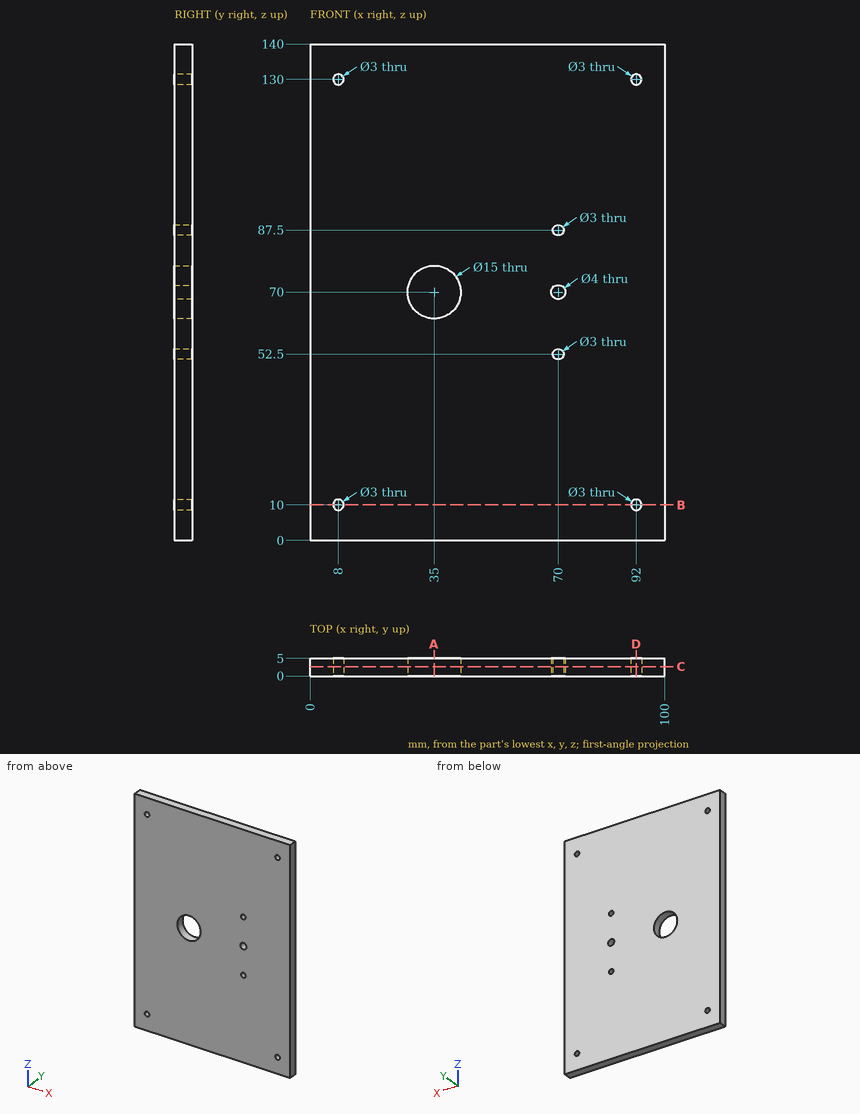
Geometry check sheet. Reference: drawing and pictorial views, mm from the part's lowest x, y, z. Coordinates: 2 decimals unless noted, no trailing zeros. Loops run counter-clockwise (first coordinate to the right, second up) from the corner with the lowest first, then second, coordinate; pieces in that order, holes last.
1) Sectioned sample at B-B (z = 10). Record the boundary of the cut face in (x, y).
2) Sectioned sample at D-D (x = 92). Record the boundary of the cut face in (y, z).
3) Sectioned sample at A-A (x = 35). Record the boundary of the cut face in (y, z).
4) Material ranges on probe 1 along Z at (x, y) = (70, 3.85); probe 2 along X at (y, z) = (2.4, 130); probe 3 along X at (y, z) = (3.15, 70), recorded low to high.
5) Sectioned sample at C-C (y = 2.65). Count the separate pieces of the cut face and the enclosed holes in it, and give its area (3 significant figures).
Check sheet entries:
1. outline: (0, 0) - (6.5, 0) - (6.5, 5) - (0, 5) - close; (9.5, 0) - (90.5, 0) - (90.5, 5) - (9.5, 5) - close; (93.5, 0) - (100, 0) - (100, 5) - (93.5, 5) - close
2. outline: (0, 0) - (5, 0) - (5, 8.5) - (0, 8.5) - close; (0, 11.5) - (5, 11.5) - (5, 128.5) - (0, 128.5) - close; (0, 131.5) - (5, 131.5) - (5, 140) - (0, 140) - close
3. outline: (0, 0) - (5, 0) - (5, 62.5) - (0, 62.5) - close; (0, 77.5) - (5, 77.5) - (5, 140) - (0, 140) - close
4. probe 1: z = 0 to 51, 54 to 68, 72 to 86, 89 to 140
4. probe 2: x = 0 to 6.5, 9.5 to 90.5, 93.5 to 100
4. probe 3: x = 0 to 27.5, 42.5 to 68, 72 to 100
5. separate pieces: 1
5. enclosed holes: 8
5. area: 13,800 mm2
